Verification items for the finished model (mm, model axes). A direction names the side the tool comes from. Coordinates: 2 decimals unless noted, no trailing zeros. Loops run counter-clockwise (first coordinate to the right, second up) from the corner with the lowest first, then second, coordinate; pieces in that order, holes last. Notation, with made-up numbers: (-33.75, 68) -> (9.25, 68) arc R20 ccw to (9.25, 85) -> close; hole circle Ø8 at (74.5, 65.5). An arc over 180 degrees is marked (long way). Answer as a JSON object with one key per item and string values. Group by question number.
Q1. Gauge pin test, flat end, axial feed: pin 1 Ø5 at (y, z) = (11, 15.5) entering from -X. Record the tip position at first contact, or that the pin passes through.
Q2. Cross-section at C-C on x = 21. Record the boundary of the cut face in (y, z), and give its area (3 significant figures).
Q3. Cross-section at A-A on x = 44. Record the boundary of the cut face in (y, z).
Q4. Set-up check for faces 1 (the flat face through (7, 9, 6)), 2 (the cylindrical face through (37.196, 7.335, 17.521)), 3 (the flat face through (23, 6, 10)), 4 (the flat face through (47, 8.5, 3)), 5 (the flat face through (21, 3, 6)): record each of +Z, -Z, +X, -X, +Y, -Y from which the full face is reachable in a straight line by a thin tool's end or side.
Q5. Cross-section at D-D on z = 14.75. Record the boundary of the cut face in (x, y).
Q6. Release check for a two-part mould opening along X. For faces 6 (the flat face through (27, 0, 7)), 7 (the cylindrical face through (4, 6, 3)) record: released by +X, released by -X, zero draft, split by the parting line, or undercut.
Q7. Scan lines: L1, parallel to Z at x = 32, y = 3.75; L2, parallel to Z at x = 16, y = 11.5; L3, parallel to Y at x = 30.35, z = 17.6. Record each from-to range of solid material in increasing order.
Q8. Cross-section at B-B on z = 7.25. Record the boundary of the cut face in (x, y).
```python
from build123d import *

# Parameters (mm, degrees)
SKETCH2_W           = 55
SKETCH2_H           = 12
BOSS_EXTRUDE1_DEPTH = 6
SKETCH3_W           = 25
SKETCH3_H           = 12
BOSS_EXTRUDE2_DEPTH = 13
SKETCH4_R           = 4.25
CUT_EXTRUDE2_DEPTH  = 30
SKETCH5_W           = 20.513890507
SKETCH5_H           = 7
CUT_EXTRUDE3_DEPTH  = 5
SKETCH6_R           = 1.6
CUT_EXTRUDE4_DEPTH  = 11
CUT_EXTRUDE5_DEPTH  = 3
SKETCH8_R           = 0.75
CUT_EXTRUDE6_DEPTH  = 3


with BuildPart() as part:
    # Sketch2 → Boss-Extrude1 (new body)
    with BuildSketch(Plane.XY):
        with Locations((27.5, 6)):
            Rectangle(SKETCH2_W, SKETCH2_H)
        with BuildLine():
            Line((6.5, 8.5), (9.5, 8.5))
            ThreePointArc((9.5, 8.5), (12, 6), (9.5, 3.5))
            Line((9.5, 3.5), (6.5, 3.5))
            ThreePointArc((6.5, 3.5), (4, 6), (6.5, 8.5))
        make_face(mode=Mode.SUBTRACT)
        with BuildLine():
            Line((48.5, 8.5), (45.5, 8.5))
            ThreePointArc((45.5, 8.5), (43, 6), (45.5, 3.5))
            Line((45.5, 3.5), (48.5, 3.5))
            ThreePointArc((48.5, 3.5), (51, 6), (48.5, 8.5))
        make_face(mode=Mode.SUBTRACT)
    extrude(amount=BOSS_EXTRUDE1_DEPTH)

    # Sketch3 → Boss-Extrude2 (add)
    with BuildSketch(Plane.XY.offset(6)):
        with Locations((27.5, 6)):
            Rectangle(SKETCH3_W, SKETCH3_H)
    extrude(amount=BOSS_EXTRUDE2_DEPTH)

    # Sketch4 → Cut-Extrude2 (cut)
    with BuildSketch(Plane.XZ):
        with BuildLine():
            ThreePointArc((27.86932209, 10), (27.75, 11), (27.86932209, 12))
            Line((27.86932209, 12), (15, 12))
            Line((15, 12), (15, 10))
            Line((15, 10), (27.86932209, 10))
        make_face()
        with Locations((32, 11)):
            Circle(SKETCH4_R)
    extrude(amount=-CUT_EXTRUDE2_DEPTH, mode=Mode.SUBTRACT)

    # Sketch5 → Cut-Extrude3 (cut)
    with BuildSketch(Plane(origin=(0, 0, 0), x_dir=(-1, 0, 0), z_dir=(0, 0, -1))):
        with Locations((-27.415473723, 6)):
            Rectangle(SKETCH5_W, SKETCH5_H)
    extrude(amount=-CUT_EXTRUDE3_DEPTH, mode=Mode.SUBTRACT)

    # Sketch6 → Cut-Extrude4 (cut)
    with BuildSketch(Plane.XY.offset(19)):
        with Locations((21, 6)):
            Circle(SKETCH6_R)
    extrude(amount=-CUT_EXTRUDE4_DEPTH, mode=Mode.SUBTRACT)

    # Sketch7 → Cut-Extrude5 (cut)
    with BuildSketch(Plane(origin=(0, 0, 5), x_dir=(-1, 0, 0), z_dir=(0, 0, -1))):
        Polygon((-17.535898385, 6), (-19.267949192, 9), (-22.732050808, 9), (-24.464101615, 6), (-22.732050808, 3), (-19.267949192, 3), align=None)
    extrude(amount=-CUT_EXTRUDE5_DEPTH, mode=Mode.SUBTRACT)

    # Sketch8 → Cut-Extrude6 (cut)
    with BuildSketch(Plane.XY.offset(19)):
        with Locations((36.85, 8)):
            Circle(SKETCH8_R)
        with Locations((30.35, 8)):
            Circle(SKETCH8_R)
    extrude(amount=-CUT_EXTRUDE6_DEPTH, mode=Mode.SUBTRACT)


solid = part.part
```
Computed values:
{
 "1": {"pin 1": "stops at x = 15"},
 "2": {"outline": "(0, 0) -> (2.5, 0) -> (2.5, 5) -> (3, 5) -> (3, 8) -> (4.4, 8) -> (4.4, 10) -> (0, 10) -> close; (0, 12) -> (4.4, 12) -> (4.4, 19) -> (0, 19) -> close; (7.6, 8) -> (9, 8) -> (9, 5) -> (9.5, 5) -> (9.5, 0) -> (12, 0) -> (12, 10) -> (7.6, 10) -> close; (7.6, 12) -> (12, 12) -> (12, 19) -> (7.6, 19) -> close", "area": "122 mm²"},
 "3": {"outline": "(0, 0) -> (4, 0) -> (4, 6) -> (0, 6) -> close; (8, 0) -> (12, 0) -> (12, 6) -> (8, 6) -> close"},
 "4": {"face 1": "+Z, -X, +Y, -Y", "face 2": "+Z", "face 3": "-X, +Y, -Y", "face 4": "+Z, -Z", "face 5": "-Z"},
 "5": {"outline": "(15, 0) -> (30, 0) -> (30, 12) -> (15, 12) -> close; (34, 0) -> (40, 0) -> (40, 12) -> (34, 12) -> close; hole circle Ø3.2 at (21, 6)"},
 "6": {"face 6": "zero draft", "face 7": "undercut"},
 "7": {"L1": "z = 5 to 6.75, 15.25 to 19", "L2": "z = 0 to 10, 12 to 19", "L3": "y = 0 to 7.25, 8.75 to 12"},
 "8": {"outline": "(15, 0) -> (30, 0) -> (30, 12) -> (15, 12) -> close; (34, 0) -> (40, 0) -> (40, 12) -> (34, 12) -> close; hole (17.54, 6) -> (19.27, 3) -> (22.73, 3) -> (24.46, 6) -> (22.73, 9) -> (19.27, 9) -> close"}
}
